Here's the drawing with two shaded views (mm, measured from the low corner). I have some questions. Round coordinates to 2 decimals unless told otherwise and drop trailing zeros. Loops run counter-clockwise (first coordinate to the right, second up) from the corner with the lowest first, then second, coordinate; pieces in that order, holes last.
(1) I want a section at C-C on y = 3.5. Write out the boundary of the cut face in (x, z).
(2) I want a section at D-D on x = 14.25. Write out the boundary of the cut face in (y, z), plus the area to 3 significant figures.
(3) Thinking about a two-plate mould opening in X: for the marked faces 1, 2 and 3, which applies, released by +X, released by -X, zero draft, split by the parting line, or undercut?
(4) If I drill on line 1 along Z through (x, y) = (13.5, 2.15); line 2 along X through (y, z) = (1.9, 0.85); line 3 along X through (y, z) = (3.45, 1.8), over which ranges is the centre line in solid material (lowest first)?
(5) I want a section at A-A on z = 1.5. Write out the boundary of the cut face in (x, y).
(6) I want a section at B-B on x = 1.5. Write out the boundary of the cut face in (y, z).
(7) Will this pin go through, and if not, where does the flat tip stop? pin 1 Ø1.6 at (x, z) = (13.5, 1.5) entering from +Y.
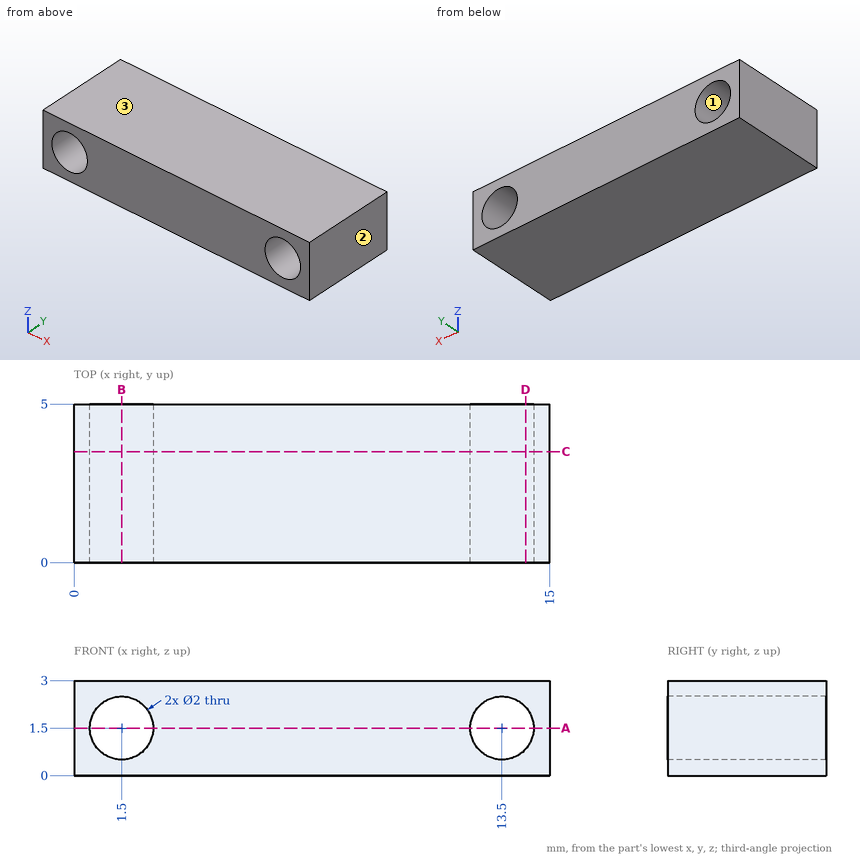
Filled sheet:
1. outline: (0, 0) - (15, 0) - (15, 3) - (0, 3) - close; hole circle Ø2 at (1.5, 1.5); hole circle Ø2 at (13.5, 1.5)
2. outline: (0, 0) - (5, 0) - (5, 0.84) - (0, 0.84) - close; (0, 2.16) - (5, 2.16) - (5, 3) - (0, 3) - close
2. area: 8.39 mm2
3. face 1: undercut
3. face 2: released by +X
3. face 3: zero draft
4. line 1: z = 0 to 0.5, 2.5 to 3
4. line 2: x = 0 to 0.74, 2.26 to 12.74, 14.26 to 15
4. line 3: x = 0 to 0.55, 2.45 to 12.55, 14.45 to 15
5. outline: (0, 0) - (0.5, 0) - (0.5, 5) - (0, 5) - close; (2.5, 0) - (12.5, 0) - (12.5, 5) - (2.5, 5) - close; (14.5, 0) - (15, 0) - (15, 5) - (14.5, 5) - close
6. outline: (0, 0) - (5, 0) - (5, 0.5) - (0, 0.5) - close; (0, 2.5) - (5, 2.5) - (5, 3) - (0, 3) - close
7. pin 1: passes through
